```python
from build123d import *

# Parameters (mm, degrees)
SKETCH1_W               = 241.3
SKETCH1_H               = 50.8
BOSS_EXTRUDE1_DEPTH     = 6.35
F_1_2_13_TAPPED_HOLE1_D = 10.71626


# Read off the part's stored shape, not the designer's step: CSK for 1/4 Flat Head Machine Screw1
with BuildPart() as part:
    # Sketch1 → Boss-Extrude1 (new body)
    with BuildSketch(Plane(origin=(0, 0, 0), x_dir=(1, 0, 0), z_dir=(0, 1, 0))):
        Rectangle(SKETCH1_W, SKETCH1_H)
    extrude(amount=BOSS_EXTRUDE1_DEPTH)

    # CSK for 1/4 Flat Head Machine Screw1 out → CSK for 1/4 Flat Head Machine Screw1 (revolve, cut)
    with BuildSketch(Plane(origin=(76.2, 0, 12.7), x_dir=(1, 0, 0), z_dir=(0, 0, 1))):
        Polygon((0, 0), (3.3782, 0), (3.3782, 2.829067416), (6.4389, 6.35), (0, 6.35), align=None)
    revolve(axis=Axis((76.2, 0, 12.7), (0, 1, 0)), mode=Mode.SUBTRACT)

    # CSK for 1_4 Flat Head Machine Screw1 2 o → CSK for 1_4 Flat Head Machine Screw1 2 (revolve, cut)
    with BuildSketch(Plane(origin=(50.8, 0, -12.7), x_dir=(1, 0, 0), z_dir=(0, 0, 1))):
        Polygon((0, 0), (3.3782, 0), (3.3782, 2.829067416), (6.4389, 6.35), (0, 6.35), align=None)
    revolve(axis=Axis((50.8, 0, -12.7), (0, 1, 0)), mode=Mode.SUBTRACT)

    # CSK for 1_4 Flat Head Machine Screw1 3 o → CSK for 1_4 Flat Head Machine Screw1 3 (revolve, cut)
    with BuildSketch(Plane(origin=(50.8, 0, 12.7), x_dir=(1, 0, 0), z_dir=(0, 0, 1))):
        Polygon((0, 0), (3.3782, 0), (3.3782, 2.829067416), (6.4389, 6.35), (0, 6.35), align=None)
    revolve(axis=Axis((50.8, 0, 12.7), (0, 1, 0)), mode=Mode.SUBTRACT)

    # CSK for 1_4 Flat Head Machine Screw1 4 o → CSK for 1_4 Flat Head Machine Screw1 4 (revolve, cut)
    with BuildSketch(Plane(origin=(76.2, 0, -12.7), x_dir=(1, 0, 0), z_dir=(0, 0, 1))):
        Polygon((0, 0), (3.3782, 0), (3.3782, 2.829067416), (6.4389, 6.35), (0, 6.35), align=None)
    revolve(axis=Axis((76.2, 0, -12.7), (0, 1, 0)), mode=Mode.SUBTRACT)

    # CSK for 1_4 Flat Head Machine Screw1 5 o → CSK for 1_4 Flat Head Machine Screw1 5 (revolve, cut)
    with BuildSketch(Plane(origin=(-50.8, 0, 12.7), x_dir=(1, 0, 0), z_dir=(0, 0, 1))):
        Polygon((0, 0), (3.3782, 0), (3.3782, 2.829067416), (6.4389, 6.35), (0, 6.35), align=None)
    revolve(axis=Axis((-50.8, 0, 12.7), (0, 1, 0)), mode=Mode.SUBTRACT)

    # CSK for 1_4 Flat Head Machine Screw1 6 o → CSK for 1_4 Flat Head Machine Screw1 6 (revolve, cut)
    with BuildSketch(Plane(origin=(-76.2, 0, -12.7), x_dir=(1, 0, 0), z_dir=(0, 0, 1))):
        Polygon((0, 0), (3.3782, 0), (3.3782, 2.829067416), (6.4389, 6.35), (0, 6.35), align=None)
    revolve(axis=Axis((-76.2, 0, -12.7), (0, 1, 0)), mode=Mode.SUBTRACT)

    # CSK for 1_4 Flat Head Machine Screw1 7 o → CSK for 1_4 Flat Head Machine Screw1 7 (revolve, cut)
    with BuildSketch(Plane(origin=(-76.2, 0, 12.7), x_dir=(1, 0, 0), z_dir=(0, 0, 1))):
        Polygon((0, 0), (3.3782, 0), (3.3782, 2.829067416), (6.4389, 6.35), (0, 6.35), align=None)
    revolve(axis=Axis((-76.2, 0, 12.7), (0, 1, 0)), mode=Mode.SUBTRACT)

    # CSK for 1_4 Flat Head Machine Screw1 8 o → CSK for 1_4 Flat Head Machine Screw1 8 (revolve, cut)
    with BuildSketch(Plane(origin=(-50.8, 0, -12.7), x_dir=(1, 0, 0), z_dir=(0, 0, 1))):
        Polygon((0, 0), (3.3782, 0), (3.3782, 2.829067416), (6.4389, 6.35), (0, 6.35), align=None)
    revolve(axis=Axis((-50.8, 0, -12.7), (0, 1, 0)), mode=Mode.SUBTRACT)

    # CSK for 1_4 Flat Head Machine Screw1 9 o → CSK for 1_4 Flat Head Machine Screw1 9 (revolve, cut)
    with BuildSketch(Plane(origin=(12.7, 0, 12.7), x_dir=(1, 0, 0), z_dir=(0, 0, 1))):
        Polygon((0, 0), (3.3782, 0), (3.3782, 2.829067416), (6.4389, 6.35), (0, 6.35), align=None)
    revolve(axis=Axis((12.7, 0, 12.7), (0, 1, 0)), mode=Mode.SUBTRACT)

    # CSK for 1_4 Flat Head Machine Screw1 11 → CSK for 1_4 Flat Head Machine Screw1 10 (revolve, cut)
    with BuildSketch(Plane(origin=(-12.7, 0, -12.7), x_dir=(1, 0, 0), z_dir=(0, 0, 1))):
        Polygon((0, 0), (3.3782, 0), (3.3782, 2.829067416), (6.4389, 6.35), (0, 6.35), align=None)
    revolve(axis=Axis((-12.7, 0, -12.7), (0, 1, 0)), mode=Mode.SUBTRACT)

    # CSK for 1_4 Flat Head Machine Screw1 13 → CSK for 1_4 Flat Head Machine Screw1 12 (revolve, cut)
    with BuildSketch(Plane(origin=(-12.7, 0, 12.7), x_dir=(1, 0, 0), z_dir=(0, 0, 1))):
        Polygon((0, 0), (3.3782, 0), (3.3782, 2.829067416), (6.4389, 6.35), (0, 6.35), align=None)
    revolve(axis=Axis((-12.7, 0, 12.7), (0, 1, 0)), mode=Mode.SUBTRACT)

    # CSK for 1_4 Flat Head Machine Screw1 15 → CSK for 1_4 Flat Head Machine Screw1 14 (revolve, cut)
    with BuildSketch(Plane(origin=(12.7, 0, -12.7), x_dir=(1, 0, 0), z_dir=(0, 0, 1))):
        Polygon((0, 0), (3.3782, 0), (3.3782, 2.829067416), (6.4389, 6.35), (0, 6.35), align=None)
    revolve(axis=Axis((12.7, 0, -12.7), (0, 1, 0)), mode=Mode.SUBTRACT)

    # 1/2-13 Tapped Hole1 (through all)
    with Locations(Plane(origin=(0, 6.35, 0), x_dir=(1, 0, 0), z_dir=(0, 1, 0))):
        with Locations((-107.95, 0), (107.95, 0)):
            Hole(F_1_2_13_TAPPED_HOLE1_D / 2)


solid = part.part
```
CAD build for the part. Positions are in the model's coordinates, mm. Round coordinates to 2 decimals unless told otherwise and drop trailing zeros. Order: outer loops, then holes, each group sorted by start corner. A loop starts at its lowest first (then second) coordinate and runs counter-clockwise, first axis right, second up.
Q1. Drop flat-ended pins along their axis: pin 1 (6 mm diameter, centred on x = -76.2, z = -12.7, fed in from -Y); pin 2 (8 mm diameter, centred on x = 76.2, z = -12.7, fed in from +Y). Give the stop position or say it passes through.
Q2. Slice it at C-C (z = 12.7). State how many separate pieces and enclosed holes the cut face has, and give its area (3 significant figures).
Q3. Slice it at B-B (x = -107.95). Write the cut outline in (y, z), and give its area (3 significant figures).
Q4. Wall check: L1, parallel to Z at x = -76.2, y = 1.15; L2, parallel to Z at x = 107.95, y = 2.75; L3, parallel to X at y = 3.5, z = -2. Give the ranges that are in metal, low to high.
Q5. Slice it at A-A (x = 12.7). Write the cut outline in (y, z).
Q6. Two-plate mould, pull along Z, no slides. Class faces 1 (the conical face through (-74.553, 3.049, -9.533)), 2 (the flat face through (120.65, 3, 0)), 3 (the flat face through (-2, 3, 25.4)): pulls with the +Z half, pulls with the -Z half, needs draft (parallel to the pull), parting line crosses it, or undercut.
Results below:
1. pin 1: passes through
1. pin 2: stops at y = 3.54
2. separate pieces: 7
2. enclosed holes: 0
2. area: 1,210 mm2
3. outline: (0, -25.4) - (6.35, -25.4) - (6.35, -5.36) - (0, -5.36) - close; (0, 5.36) - (6.35, 5.36) - (6.35, 25.4) - (0, 25.4) - close
3. area: 255 mm2
4. L1: z = -25.4 to -16.08, -9.32 to 9.32, 16.08 to 25.4
4. L2: z = -25.4 to -5.36, 5.36 to 25.4
4. L3: x = -120.65 to -112.92, -102.98 to 102.98, 112.92 to 120.65
5. outline: (0, -25.4) - (6.35, -25.4) - (6.35, -19.14) - (2.83, -16.08) - (0, -16.08) - close; (0, -9.32) - (2.83, -9.32) - (6.35, -6.26) - (6.35, 6.26) - (2.83, 9.32) - (0, 9.32) - close; (0, 16.08) - (2.83, 16.08) - (6.35, 19.14) - (6.35, 25.4) - (0, 25.4) - close
6. face 1: undercut
6. face 2: needs draft
6. face 3: pulls with the +Z half
